```python
from build123d import *

# Parameters (mm, degrees)
F0_W     = 20
F0_H     = 20
F1_DEPTH = 2.5
F2_R     = 2.49999


# Not quite as in the source:
# - a fillet or chamfer is up to 0.001 mm smaller than in the source, because OpenCascade refuses the exact size


with BuildPart() as f1:
    # F0 (on Top) → F1 (new body)
    with BuildSketch(Plane.XY):
        Rectangle(F0_W, F0_H)
    extrude(amount=F1_DEPTH)

    # F2 (radius 2.5 in the source; OpenCascade refuses exactly that, so slightly less here)
    f2_edges = [f1.edges().sort_by_distance(p)[0] for p in [
        (10, -10, 1.25),
        (10, 10, 1.25),
        (-10, -10, 1.25),
        (-10, 10, 1.25),
        (0, -10, 2.5),
        (10, 0, 2.5),
        (0, 10, 2.5),
        (-10, 0, 2.5),
    ]]
    fillet(f2_edges, radius=F2_R)


solid = f1.part
```
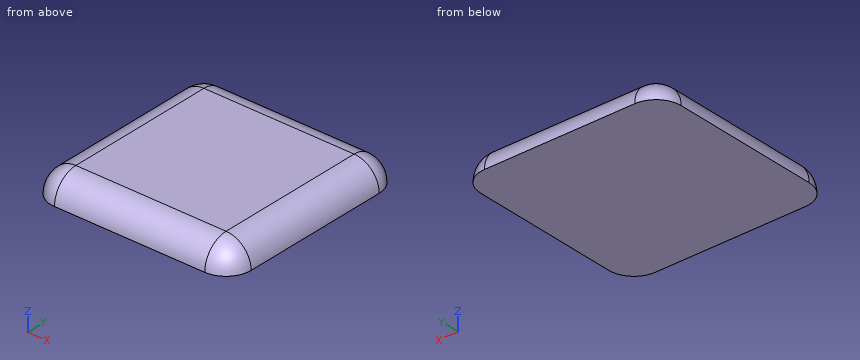
Model file for the job. Use its own axes, mm. Coordinates: 2 decimals unless noted, no trailing zeros. Order: outer loops, then holes, each group sorted by start corner. A loop starts at its lowest first (then second) coordinate and runs counter-clockwise, first axis right, second up. Notation, with made-up numbers: (17, 79.5) -> (52, 79.5) arc R10 ccw to (52, 98.5) -> close; hole circle Ø10 at (-18.75, -29). An arc over 180 degrees is marked (long way). Answer as a JSON object with one key per item and string values. Group by question number.
1) Flat gauge pins, fed straight in: pin 1 (1.5 mm diameter, centred on x = -3.5, z = 1.5, fed in from -Y); pin 2 (1 mm diameter, centred on y = 2.5, z = 1.5, fed in from -X). Where does each tip first touch, or does it go through?
2) Cut at C-C, the plane z = 1.9. Write the cut outline in (x, y).
3) Cut at D-D, the plane z = 0.3. Write the cut outline in (x, y).
4) Drill centre lines: L1, parallel to Y at x = 2.75, z = 0.5; L2, parallel to X at y = 6.5, z = 1; L3, parallel to Y at x = 6.5, z = 1.85. Where is each one in solid material? Low to high.
Check values:
{
 "1": {"pin 1": "stops at y = -9.88", "pin 2": "stops at x = -9.79"},
 "2": {"outline": "(-9.12, -7.5) arc R1.62 ccw to (-7.5, -9.12) -> (7.5, -9.12) arc R1.62 ccw to (9.12, -7.5) -> (9.12, 7.5) arc R1.62 ccw to (7.5, 9.12) -> (-7.5, 9.12) arc R1.62 ccw to (-9.12, 7.5) -> close"},
 "3": {"outline": "(-9.98, -7.5) arc R2.48 ccw to (-7.5, -9.98) -> (7.5, -9.98) arc R2.48 ccw to (9.98, -7.5) -> (9.98, 7.5) arc R2.48 ccw to (7.5, 9.98) -> (-7.5, 9.98) arc R2.48 ccw to (-9.98, 7.5) -> close"},
 "4": {"L1": "y = -9.95 to 9.95", "L2": "x = -9.79 to 9.79", "L3": "y = -9.18 to 9.18"}
}
